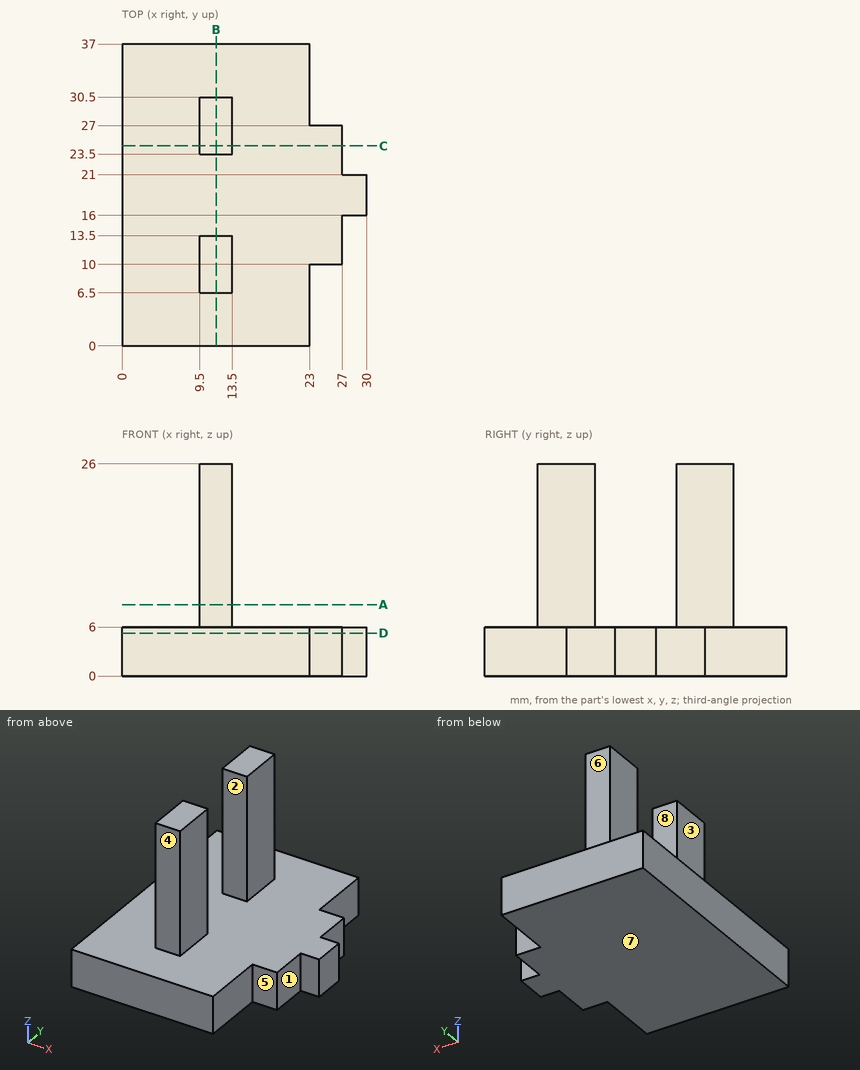
Job drawing, mm, ordinate dimensions from the low corner. One solid piece. A direction names the side the tool comes from. Give positions to 0.01 mm unless a question says otherwise; leave off trailing zeros. Loops run counter-clockwise (first coordinate to the right, second up) from the corner with the lowest first, then second, coordinate; pieces in that order, holes last. Notation, with made-up numbers: (4.5, 73.5) - (52.5, 73.5) arc R22 ccw to (52.5, 111.5) - close; hole circle Ø2 at (14.5, 4). An arc over 180 degrees is marked (long way). Use one line per item in the form item = value.
(1) Drop flat-ended pins along their axis: P1, Ø8, axis at y = 10.5, z = 15.5, coming from the -X side; P2, Ø2.5, axis at x = 28, z = 4, coming from the -Y side; P3, Ø6.5, axis at y = 32, z = 2, coming from the +X side; P4, Ø12, axis at x = 22.5, z = 3, coming from the -Y side. Give the stop position or say it passes through.
Determined:
P1 = 9.5
P2 = 10
P3 = 23
P4 = 0
(2) Drill centre lines: L1, parallel to Y at x = 11.25, z = 18.75; L2, parallel to X at y = 12, z = 14; L3, parallel to Z at x = 18.25, y = 22. Where is each one in solid material? Low to high.
Determined:
L1 = 6.5 to 13.5, 23.5 to 30.5
L2 = 9.5 to 13.5
L3 = 0 to 6
(3) Cut at C-C (y = 24.5). Give the cut face in (x, z), then the cut area to 3 significant figures.
Determined:
outline = (0, 0) - (27, 0) - (27, 6) - (13.5, 6) - (13.5, 26) - (9.5, 26) - (9.5, 6) - (0, 6) - close
area = 242 mm^2
(4) Pull direction Y, two halves, no side cores. Call the marked faces 5, 6, 7 and 8: pulls with the +Y half, pulls with the -Y half, needs draft (parallel to the pull), parting line crosses it, or undercut.
Determined:
face_5 = pulls with the -Y half
face_6 = pulls with the +Y half
face_7 = needs draft
face_8 = undercut
(5) 3-axis set-ups, long thin cutter, end or side, ignore diameter. For the marked faces 1, 2, 3 and 4: which of +Z, -Z, +X, -X, +Y, -Y reach the whole face in a straight line?
Determined:
face_1 = +Z, -Z, +X, -Y
face_2 = +Z, +X, -X
face_3 = +Z, -X, +Y, -Y
face_4 = +Z, +X, -X, -Y
(6) Cut at A-A (z = 8.75). Give the cut face in (x, y), then the cut area to 3 significant figures.
Determined:
outline = (9.5, 6.5) - (13.5, 6.5) - (13.5, 13.5) - (9.5, 13.5) - close; (9.5, 23.5) - (13.5, 23.5) - (13.5, 30.5) - (9.5, 30.5) - close
area = 56.0 mm^2
(7) Cut at D-D (z = 5.25). Give the cut face in (x, y), then the cut area to 3 significant figures.
Determined:
outline = (0, 0) - (23, 0) - (23, 10) - (27, 10) - (27, 16) - (30, 16) - (30, 21) - (27, 21) - (27, 27) - (23, 27) - (23, 37) - (0, 37) - close
area = 934 mm^2
(8) Cut at B-B (x = 11.5). Give the cut face in (y, z).
Determined:
outline = (0, 0) - (37, 0) - (37, 6) - (30.5, 6) - (30.5, 26) - (23.5, 26) - (23.5, 6) - (13.5, 6) - (13.5, 26) - (6.5, 26) - (6.5, 6) - (0, 6) - close
